Could you check a few things on this drawing? It's one solid part, dimensions in mm from its lowest x, y, z. Coordinates: 2 decimals unless noted, no trailing zeros. Loops run counter-clockwise (first coordinate to the right, second up) from the corner with the lowest first, then second, coordinate; pieces in that order, holes last.
1) Thinking about a two-plate mould opening in Z: for the marked faces 1 and 2, which applies, released by +Z, released by -Z, zero draft, split by the parting line, or undercut?
2) Imagine slicing it at B-B on y = 100. Please give me the cut outline in (x, z), plus the area to 3 significant figures.
3) Imagine slicing it at A-A on x = 60. Please give me the cut outline in (y, z).
4) If I drill on line 1 along Y through (x, z) = (60, 1.3); line 2 along Y through (x, z) = (53, 3.35), over which ranges is the centre line in solid material (lowest first)?
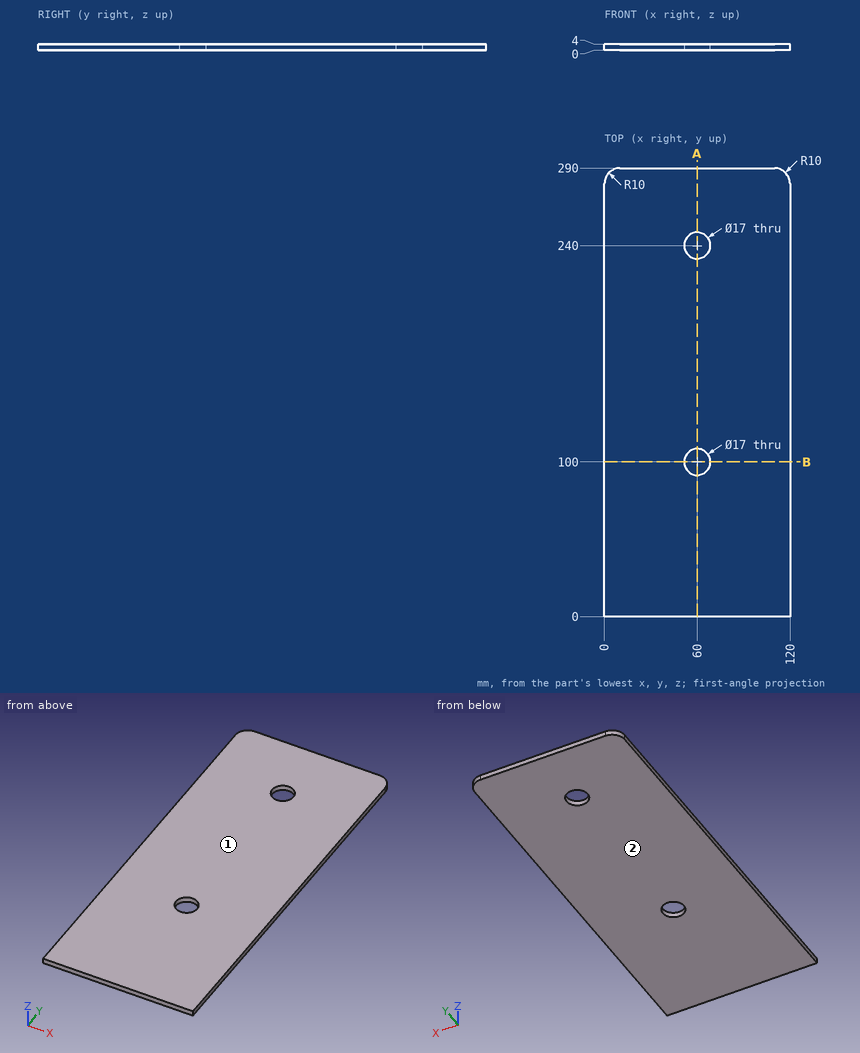
Filled in:
1. face 1: released by +Z
1. face 2: released by -Z
2. outline: (0, 0) - (51.5, 0) - (51.5, 4) - (0, 4) - close; (68.5, 0) - (120, 0) - (120, 4) - (68.5, 4) - close
2. area: 412 mm2
3. outline: (0, 0) - (91.5, 0) - (91.5, 4) - (0, 4) - close; (108.5, 0) - (231.5, 0) - (231.5, 4) - (108.5, 4) - close; (248.5, 0) - (290, 0) - (290, 4) - (248.5, 4) - close
4. line 1: y = 0 to 91.5, 108.5 to 231.5, 248.5 to 290
4. line 2: y = 0 to 95.18, 104.82 to 235.18, 244.82 to 290
